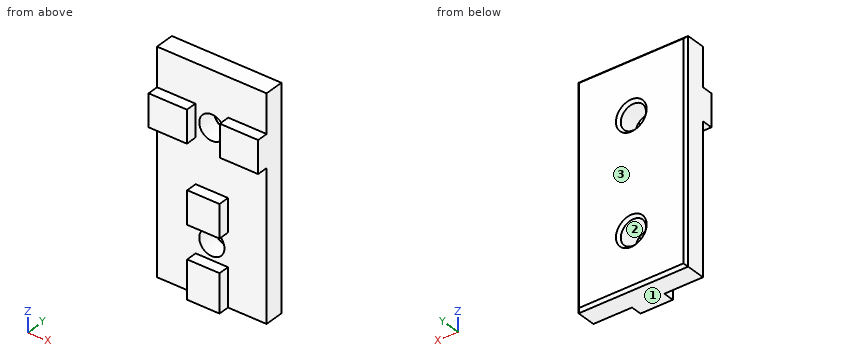
```python
from build123d import *

# Parameters (mm, degrees)
ESBO_O1_W                  = 20
ESBO_O1_H                  = 40
RESSALTO_EXTRUS_O1_DEPTH   = 4
ESBO_O2_R                  = 2.3
CORTE_EXTRUS_O1_DEPTH      = 1
CORTE_EXTRUS_O1_DEPTH_BACK = 5
ESBO_O3_W                  = 5.9
ESBO_O3_H                  = 6
ESBO_O3_H_2                = 7
ESBO_O3_W_2                = 7
ESBO_O3_H_3                = 5.9
RESSALTO_EXTRUS_O2_DEPTH   = 2
CHANFRO1_SIZE              = 0.5


with BuildPart() as part:
    # Esboço1 → Ressalto-extrusão1 (new body)
    with BuildSketch(Plane(origin=(0, 0, 0), x_dir=(1, 0, 0), z_dir=(0, 1, 0))):
        Rectangle(ESBO_O1_W, ESBO_O1_H)
    extrude(amount=RESSALTO_EXTRUS_O1_DEPTH)

    # Esboço2 → Corte-extrusão1 (cut, two sides)
    with BuildSketch(Plane(origin=(0, 4, 0), x_dir=(1, 0, 0), z_dir=(0, 1, 0))) as corte_extrus_o1_sk:
        with Locations((0, 10)):
            Circle(ESBO_O2_R)
        with Locations((0, -10)):
            Circle(ESBO_O2_R)
    extrude(amount=CORTE_EXTRUS_O1_DEPTH, mode=Mode.SUBTRACT)
    extrude(corte_extrus_o1_sk.sketch, amount=-CORTE_EXTRUS_O1_DEPTH_BACK, mode=Mode.SUBTRACT)

    # Esboço3 → Ressalto-extrusão2 (add)
    with BuildSketch(Plane.XZ):
        with Locations((0, -4)):
            Rectangle(ESBO_O3_W, ESBO_O3_H)
        with Locations((0, -16.5)):
            Rectangle(ESBO_O3_W, ESBO_O3_H_2)
        with Locations((-6.5, 10)):
            Rectangle(ESBO_O3_W_2, ESBO_O3_H_3)
        with Locations((6.5, 10)):
            Rectangle(ESBO_O3_W_2, ESBO_O3_H_3)
    extrude(amount=RESSALTO_EXTRUS_O2_DEPTH)

    # Chanfro1
    chanfro1_edges = [part.edges().sort_by_distance(p)[0] for p in [
        (-10, 4, 0),
        (0, 4, 20),
        (-2.3, 4, -10),
        (-2.3, 4, 10),
        (10, 4, 0),
        (0, 4, -20),
    ]]
    chamfer(chanfro1_edges, length=CHANFRO1_SIZE)


solid = part.part
```
Source: CAD feature listing. Evaluate the final solid. Frame: model axes, mm. Face numbers are marked on the shaded views. Round coordinates to 2 decimals unless told otherwise and drop trailing zeros. Loops run counter-clockwise (first coordinate to the right, second up) from the corner with the lowest first, then second, coordinate; pieces in that order, holes last.
1. Section query D-D on z = -2.5. Output: boundary loops of the cut face in (x, y).
2. Ray query, L1, parallel to Z at x = 0, y = 1.45; L2, parallel to Z at x = 0.25, y = 3.75; L3, parallel to X at y = 1.15, z = -10. Return the intervals inside material, ascending.
3. Section query C-C on y = 0.75. Output: boundary loops of the cut face in (x, z), and give its area (3 significant figures).
4. Mould query, pull axis Z, two halves, no side actions, for the marked faces 1, 2 and 3. Classes: released by +Z, released by -Z, zero draft, split by the parting line, or undercut.
5. Contact query for flat-ended pins moving along their axis: pin 1 (1 mm diameter, centred on x = -6, y = -1.5, fed in from -Z); pin 2 (1.6 mm diameter, centred on y = -1.5, z = -4, fed in from +X); pin 3 (5.5 mm diameter, centred on x = 0, z = 10, fed in from +Y); pin 4 (2 mm diameter, centred on x = -5.5, y = -0.5, fed in from +Z). Output: stop coordinate, or through.
6. Section query B-B on z = 10. Output: boundary loops of the cut face in (x, y), and give its area (3 significant figures).
7. Section query A-A on x = 0. Output: boundary loops of the cut face in (y, z).
Answers below:
1. outline: (-10, 0) - (-2.95, 0) - (-2.95, -2) - (2.95, -2) - (2.95, 0) - (10, 0) - (10, 3.5) - (9.5, 4) - (-9.5, 4) - (-10, 3.5) - close
2. L1: z = -20 to -12.3, -7.7 to 7.7, 12.3 to 20
2. L2: z = -19.75 to -12.54, -7.46 to 7.46, 12.54 to 19.75
2. L3: x = -10 to -2.3, 2.3 to 10
3. outline: (-10, -20) - (10, -20) - (10, 20) - (-10, 20) - close; hole circle Ø4.6 at (0, -10); hole circle Ø4.6 at (0, 10)
3. area: 767 mm2
4. face 1: released by -Z
4. face 2: undercut
4. face 3: zero draft
5. pin 1: stops at z = 7.05
5. pin 2: stops at x = 2.95
5. pin 3: stops at y = 3.95
5. pin 4: stops at z = 20
6. outline: (-10, -2) - (-3, -2) - (-3, 0) - (-2.3, 0) - (-2.3, 3.5) - (-2.8, 4) - (-9.5, 4) - (-10, 3.5) - close; (2.3, 0) - (3, 0) - (3, -2) - (10, -2) - (10, 3.5) - (9.5, 4) - (2.8, 4) - (2.3, 3.5) - close
6. area: 89.1 mm2
7. outline: (-2, -20) - (3.5, -20) - (4, -19.5) - (4, -12.8) - (3.5, -12.3) - (0, -12.3) - (0, -13) - (-2, -13) - close; (-2, -7) - (0, -7) - (0, -7.7) - (3.5, -7.7) - (4, -7.2) - (4, 7.2) - (3.5, 7.7) - (0, 7.7) - (0, -1) - (-2, -1) - close; (0, 12.3) - (3.5, 12.3) - (4, 12.8) - (4, 19.5) - (3.5, 20) - (0, 20) - close
